The drawing under review shows one solid part. Ordinate dimensions are in mm from its lowest x, y, z. Coordinates: 2 decimals unless noted, no trailing zeros. Write each loop counter-clockwise with the first axis right and the second up, starting at its lowest first coordinate (ties: lowest second). Pieces come first, ordered by that corner, then holes. Notation, with made-up numbers: (79.25, 86.5) -> (95.25, 86.5) arc R14 cw to (95.25, 109.5) -> close; hole circle Ø4 at (-16, 14). An arc over 180 degrees is marked (long way). One line per item, written item: value. Start each with the question number.
1) For probe 1 along Y at (x, z) = (3.75, 20); probe 2 along Y at (x, z) = (4.25, 17); probe 3 along Z at (x, y) = (1, 22), list the stretches that pass through material, from the lowest coordinate up. Write a range as from..to.
2) Add section B-B (y = 102.5). State the section outline as (x, z) points, and give its area (3 significant figures).
3) Add section C-C (x = 3.25). State the section outline as (y, z) points.
4) Mouldability with a two-part tool opening along Y and no side actions: class the marked faces 1, 2 and 3 as released by +Y, released by -Y, zero draft, split by the parting line, or undercut.
5) Add section A-A (z = 20). State the section outline as (x, y) points.
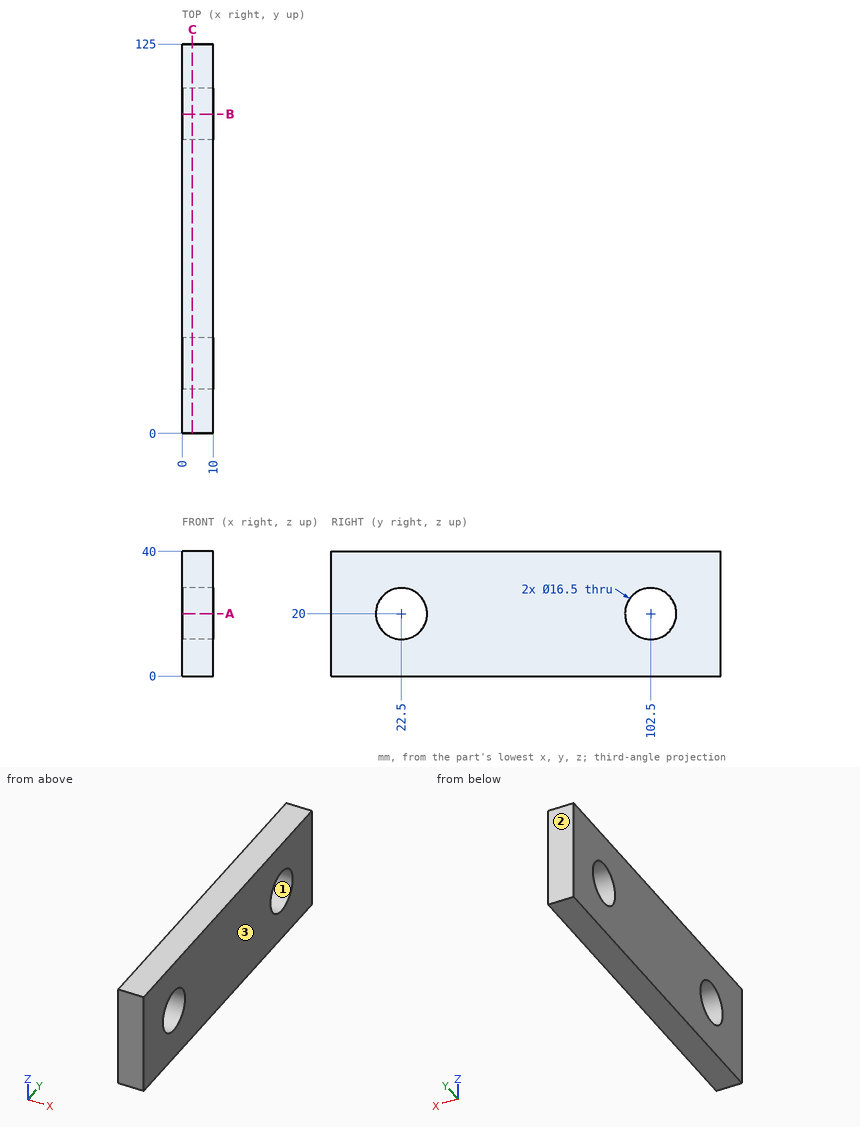
Numbers:
1. probe 1: 0..14.25, 30.75..94.25, 110.75..125
1. probe 2: 0..14.81, 30.19..94.81, 110.19..125
1. probe 3: 0..11.77, 28.23..40
2. outline: (0, 0) -> (10, 0) -> (10, 11.75) -> (0, 11.75) -> close; (0, 28.25) -> (10, 28.25) -> (10, 40) -> (0, 40) -> close
2. area: 235 mm²
3. outline: (0, 0) -> (125, 0) -> (125, 40) -> (0, 40) -> close; hole circle Ø16.5 at (22.5, 20); hole circle Ø16.5 at (102.5, 20)
4. face 1: undercut
4. face 2: released by +Y
4. face 3: zero draft
5. outline: (0, 0) -> (10, 0) -> (10, 14.25) -> (0, 14.25) -> close; (0, 30.75) -> (10, 30.75) -> (10, 94.25) -> (0, 94.25) -> close; (0, 110.75) -> (10, 110.75) -> (10, 125) -> (0, 125) -> close
